Study the drawing (mm; zero at the part's minimum x, y, z) and answer. Coordinates: 2 decimals unless noted, no trailing zeros. Order: outer loops, then holes, each group sorted by start corner. A loop starts at its lowest first (then second) coordinate and runs counter-clockwise, first axis right, second up. Notation, with made-up numbers: (89, 11.25) -> (120, 11.25) arc R28 ccw to (120, 36.25) -> close; hole circle Ø8 at (44.5, -12.5). An arc over 180 degrees is marked (long way). Write each question's results on one line, items separated by ' | '. Start each with the question number.
(1) The part is cut by section D-D, the plane z = 14. Give the vertices of the cut face in (x, y), then the cut area to 3 significant figures.
(2) Determine the mould class of the marked faces 1, 2, 3 and 4 for opening direction X: +X half, -X half, draft (parallel to the pull), parting line (faces both ways), or undercut.
(3) The part is cut by section B-B, the plane y = 2.45. Give the vertices of the cut face in (x, z).
(4) Straight lines are drawn through the part: L1, parallel to Y at x = 2.65, z = 3.25; L2, parallel to Z at x = 1.3, y = 3.2; L3, parallel to Z at x = 3.4, y = 1.1. For each, find the intervals that lie inside material, in ascending order.
(5) The part is cut by section A-A, the plane z = 2.5. Give the vertices of the cut face in (x, y).
(6) The part is cut by section C-C, the plane x = 2.35. Give the vertices of the cut face in (y, z), then the cut area to 3 significant figures.
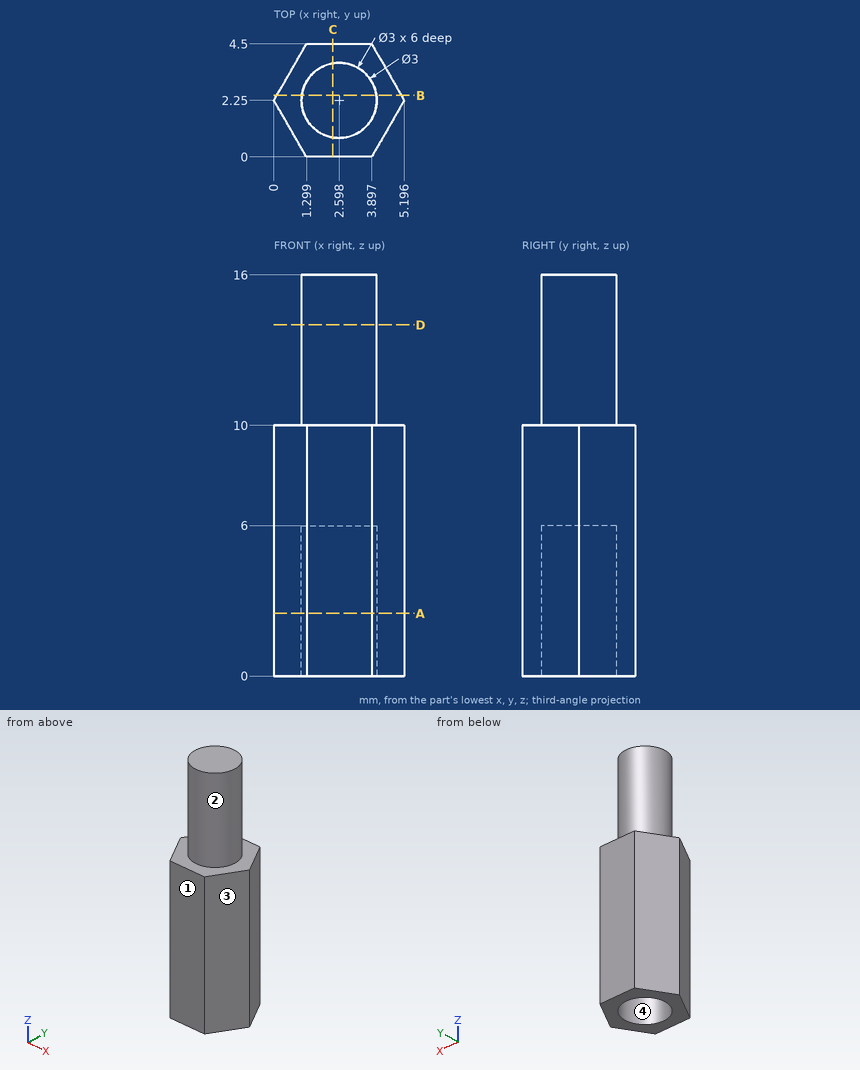
Established:
1) outline: circle Ø3 at (2.6, 2.25) | area: 7.07 mm^2
2) face 1: draft | face 2: parting line | face 3: +X half | face 4: undercut
3) outline: (0.12, 0) -> (1.11, 0) -> (1.11, 6) -> (4.08, 6) -> (4.08, 0) -> (5.08, 0) -> (5.08, 10) -> (4.08, 10) -> (4.08, 16) -> (1.11, 16) -> (1.11, 10) -> (0.12, 10) -> close
4) L1: y = 0 to 0.75, 3.75 to 4.5 | L2: z = 0 to 10 | L3: z = 6 to 16
5) outline: (0, 2.25) -> (1.3, 0) -> (3.9, 0) -> (5.2, 2.25) -> (3.9, 4.5) -> (1.3, 4.5) -> close; hole circle Ø3 at (2.6, 2.25)
6) outline: (0, 0) -> (0.77, 0) -> (0.77, 6) -> (3.73, 6) -> (3.73, 0) -> (4.5, 0) -> (4.5, 10) -> (3.73, 10) -> (3.73, 16) -> (0.77, 16) -> (0.77, 10) -> (0, 10) -> close | area: 45.0 mm^2
